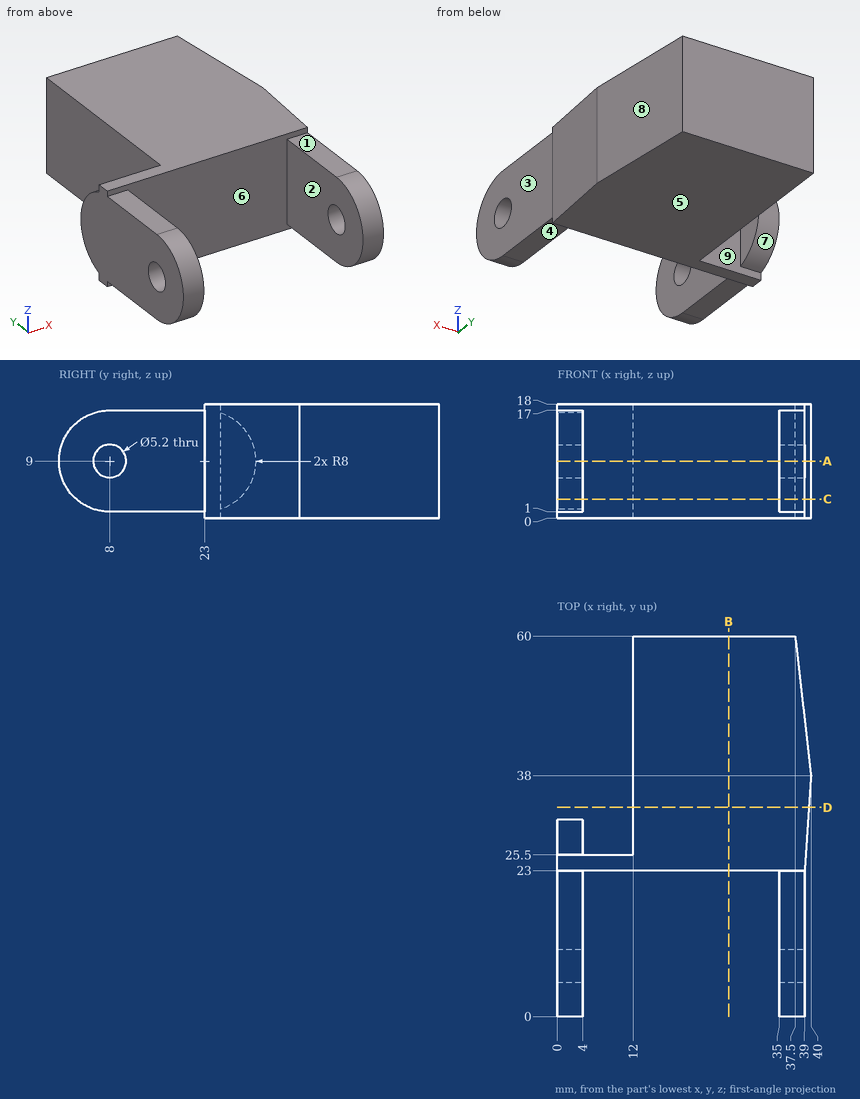
Answer from the drawing. Dimensions are ordinates in mm from the lowest x, y and z of the part. A direction names the side the tool comes from. Give positions to 0.01 mm unless a question says otherwise; leave off trailing zeros. Write each loop counter-clockwise with the first axis right and the second up, starting at its lowest first coordinate (ties: lowest second). Pieces come first, ordered by that corner, then holes. Notation, with made-up numbers: (86.5, -24) - (132.5, -24) arc R32 cw to (132.5, 6) - close; hole circle Ø2 at (-4, 64). An arc over 180 degrees is marked (long way). Answer in a Markdown table with one row per item. Add a question column.
Item 1: Section D-D, the plane y = 33 is taken. Write down the section's boundary in (x, z), and give its area (3 significant figures).
Item 2: Determine the mould class of the marked faces 6, 7, 8 and 9 for opening direction X: pulls with the +X half, pulls with the -X half, needs draft (parallel to the pull), parting line crosses it, or undercut.
Item 3: Section B-B, the plane x = 27 is taken. Write down the section's boundary in (y, z), and give its area (3 significant figures).
Item 4: A tool of negligible diameter and unlimited length cuts with its end or side. For the marked faces 1, 2, 3, 4 and 5, from which of +Z, -Z, +X, -X, +Y, -Y can it reach the whole face along a straight path? Write none if from no direction.
Item 5: Find the intervals of material crossed by L1, parallel to X at y = 14, z = 11.75; L2, parallel to Y at x = 2.8, z = 9; L3, parallel to Y at x = 37.2, z = 9, in increasing order.
Item 6: Section C-C, the plane z = 3 is taken. Write down the section's boundary in (x, y), and give its area (3 significant figures).
Item 7: Flat-ended cylindrical pins translate along their axes: P1, Ø5, axis at y = 15, z = 7, coming from the +X side; P2, Ø5.5, axis at x = 14, z = 5, coming from the -Y side; P3, Ø3, axis at y = 28, z = 9.5, coming from the +X side; P4, Ø4, axis at y = 8, z = 9, coming from the -X side. Find the tip coordinate at first contact, or state that the pin passes through.
Item 8: Section A-A, the plane z = 9 is taken. Write down the section's boundary in (x, y).
Recorded:
| question | item | result |
|---|---|---|
| 1 | outline | (12, 0) - (39.67, 0) - (39.67, 18) - (12, 18) - close |
| 1 | area | 498 mm2 |
| 2 | face 6 | undercut |
| 2 | face 7 | needs draft |
| 2 | face 8 | pulls with the +X half |
| 2 | face 9 | undercut |
| 3 | outline | (23, 0) - (60, 0) - (60, 18) - (23, 18) - close |
| 3 | area | 666 mm2 |
| 4 | face 1 | +Z, +X, -X, -Y |
| 4 | face 2 | +Z, -Z, -Y |
| 4 | face 3 | +Z, -Z, +X, -Y |
| 4 | face 4 | -Z, +X, -X, -Y |
| 4 | face 5 | -Z, +X, -X, +Y, -Y |
| 5 | L1 | x = 0 to 4, 35 to 39 |
| 5 | L2 | y = 0 to 5.4, 10.6 to 31 |
| 5 | L3 | y = 0 to 5.4, 10.6 to 60 |
| 6 | outline | (0, 2.71) - (4, 2.71) - (4, 23) - (35, 23) - (35, 2.71) - (39, 2.71) - (39, 23) - (40, 38) - (37.5, 60) - (12, 60) - (12, 25.5) - (4, 25.5) - (4, 28.29) - (0, 28.29) - close |
| 6 | area | 1,200 mm2 |
| 7 | P1 | stops at x = 39 |
| 7 | P2 | stops at y = 23 |
| 7 | P3 | stops at x = 39.43 |
| 7 | P4 | passes through |
| 8 | outline | (0, 0) - (4, 0) - (4, 5.4) - (0, 5.4) - close; (0, 10.6) - (4, 10.6) - (4, 23) - (35, 23) - (35, 10.6) - (39, 10.6) - (39, 23) - (40, 38) - (37.5, 60) - (12, 60) - (12, 25.5) - (4, 25.5) - (4, 31) - (0, 31) - close; (35, 0) - (39, 0) - (39, 5.4) - (35, 5.4) - close |
